Can you work these out from the model? Positions are in its coordinate system, mm. Face numbers are marked on the shaded views. A direction names the side the tool comes from. Round coordinates to 2 decimals unless told otherwise and drop trailing zeros. Write each loop counter-clockwise with the first axis right and the second up, starting at its lowest first coordinate (ties: lowest second). Pieces come first, ordered by that corner, then holes. Notation, with made-up numbers: M -35.75,21.5 L -23.75,21.5 A27 cw -23.75,54.5 Z; hole C 36,62.25 d3. An arc over 180 degrees is marked long. Answer as a JSON object with one key per item and string values. Group by question number.
1) On a 3-axis mill with a long thin cutter (end or side, diameter ignored), from which of +Z, -Z, +X, -X, +Y, -Y can I reach the whole of each face in a straight line? I mean the marked faces 1 and 2. Say none if no direction works.
2) Suppose I cut it at A-A, the plane z = 0. Write out the boundary of the cut face in (x, y) (3 decimals).
3) Suppose I cut it at B-B, the plane y = 0. Write out the boundary of the cut face in (x, z).
4) I'm going to push flat-ended pins straight in: pin 1 Ø4 at (x, z) = (23.5, -2.5) entering from +Y; pin 2 Ø2 at (x, z) = (-1.5, -1.5) entering from +Y; pin 3 Ø1.5 at (x, y) = (9.5, 1) entering from -Z. Where does each tip first touch, or does it pass through?
5) Please list where these lines run through material, in increasing order: L1, parallel to X at y = -2, z = 1.75; L2, parallel to Z at x = 22, y = 0; L3, parallel to X at y = 0, z = 0. Write a range as [from, to].
6) Suppose I cut it at C-C, the plane x = 16.5. Write out the boundary of the cut face in (y, z).
Autodesk Inventor part; units mm, degrees
ref_plane "Work Plane1" through (30.1625, 0, 0) normal (0, 0, -1) x (1, 0, 0)
ref_plane "YZ Plane" through (0, 0, 0) normal (1, 0, 0) x (0, 1, 0)
ref_plane "XZ Plane" through (0, 0, 0) normal (0, 1, 0) x (-1, 0, 0)
sketch "Эскиз1" plane through (0, 0, 0) normal (0, 0, 1) x (1, 0, 0)
  line L0 (-2.6, 0) -> (40, 0)
  line L1 (40, 0) -> (40, 2)
  line L2 (40, 2) -> (18, 2)
  line L3 (18, 2) -> (17.5706, 2)
  line L4 (17.5706, 2) -> (0, 2)
  line L5 (0, 2) -> (0, 3.5)
  line L6 (-11.12, 0) -> (48.52, 0)
  line L7 (0, -0.7) -> (0, 4.2)
  line L8 (-2.6, 0) -> (-2.6, 3.5)
  line L9 (0, 3.5) -> (-2.6, 3.5)
  dimension "d0" = 40
  dimension "d1" = 22
  dimension "d2" = 0.4294
  dimension "d3" = 2.6
  dimension "d4" = 4
  dimension "d5" = 4
  dimension "d9" = 7
  dimension "d10" = 0
revolve "Базовый элемент" add sketch "Эскиз1" angle 360 about axis through (-2.6, 0, 0) along (1, 0, 0)
sketch "Эскиз2" plane through (-2.6, 0, 0) normal (-1, 0, 0) x (0, 0, 1)
  circle A0 centre (0, 0) radius 3.5
  line L0 (0, 0) -> (0, 3.5)
  line L1 (-3.5, 0.455) -> (3.5, 0.455)
  line L2 (3.5, 0.455) -> (3.5, -0.455)
  line L3 (3.5, -0.455) -> (-3.5, -0.455)
  line L4 (-3.5, -0.455) -> (-3.5, 0.455)
  line L5 (-3.5, 0) -> (3.5, 0) construction
  line L6 (0, 0.455) -> (0, -0.455) construction
  dimension "d11" = 0.91
  dimension "d12" = 7
fillet "Сопряжение1" radius 0.01 1 edges at (-2.6, -3.5, 0)
extrude "Паз" cut sketch "Эскиз2" against normal blind 1.82 contours A0 L3 L1 | L2 L3 A0 | A0 L1 L2 | L3 L4 A0 | A0 L4 L1
thread "Резьба"
chamfer "Chamfer4" distance 0.4 angle 45 1 edges at (40, -2, 0)
ref_plane "Work Plane1" through (30.1625, 0, 0) normal (0, 0, -1) x (1, 0, 0)
equation "\"d11\" = SBR"
equation "\"d12\" = KOD"
equation "\"d13\" = RR"
equation "\"d16\" = STI"
equation "\"d14\" = GEL"
equation "\"d40\" = 0.1 * GD"
equation "\"d0\" = NLG"
equation "\"d1\" = GEL"
equation "\"d2\" = GAL"
equation "\"d3\" = KOH"
equation "\"d4\" = GD"
equation "\"d5\" = BDM"
equation "\"d9\" = KOD"
equation "\"GD\" = NND"
equation "\"NLG\" = 40"
equation "\"GEL\" = 22"
equation "\"KOD\" = 7"
equation "\"KOH\" = 2.6"
equation "\"GAL\" = 0.61345 * PTC"
equation "\"BDM\" = NND"
equation "\"RR\" = 0.01"
equation "\"SBR\" = 0.91"
equation "\"STI\" = 1.82"
equation "\"KEWI\" = 0"
equation "\"GUL\" = 0.61345 * PTC"
equation "\"SPD\" = NND - 1.2269 * PTC"
equation "\"PTC\" = 0.7"
equation "\"THREADDIA\" = 4"
equation "\"TOA\" = 30deg"
equation "\"FAWI\" = 45deg"
equation "\"NND\" = 4"
equation "\"GD1\" = THREADDIA - 1.2269 * PTC"
properties part number "Винт M4-6gx40 ГОСТ 1491-80" material "Сталь, мягкая"
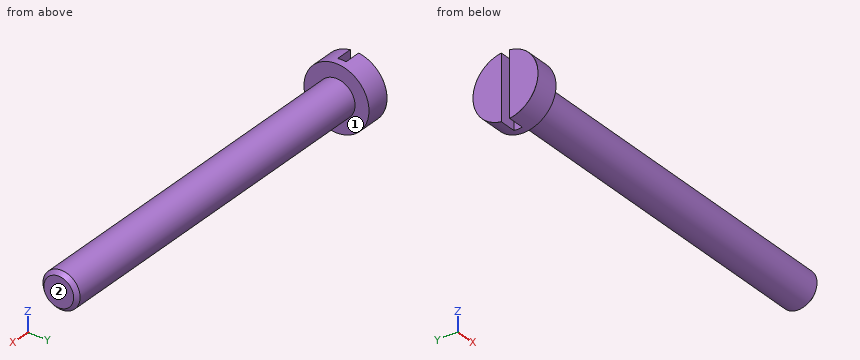
Results:
{
 "1": {"face 1": "+X", "face 2": "+Z, -Z, +X, +Y, -Y"},
 "2": {"outline": "M -2.6,-3.49 A0.01 ccw -2.59,-3.5 L 0,-3.5 L 0,-2 L 39.6,-2 L 40,-1.6 L 40,1.6 L 39.6,2 L 0,2 L 0,3.5 L -2.59,3.5 A0.01 ccw -2.6,3.49 L -2.6,0.455 L -0.78,0.455 L -0.78,-0.455 L -2.6,-0.455 Z"},
 "3": {"outline": "M -0.78,-3.5 L 0,-3.5 L 0,-2 L 39.6,-2 L 40,-1.6 L 40,1.6 L 39.6,2 L 0,2 L 0,3.5 L -0.78,3.5 Z"},
 "4": {"pin 1": "y = 1.94", "pin 2": "y = 3.46", "pin 3": "z = -1.98"},
 "5": {"L1": "[-2.6, 0]", "L2": "[-2, 2]", "L3": "[-0.78, 40]"},
 "6": {"outline": "C 0,0 d4"}
}
